For this review, use the dimensioned drawing (mm, ordinates from the lowest corner) and the shaded views. Round coordinates to 2 decimals unless told otherwise and drop trailing zeros. Loops run counter-clockwise (first coordinate to the right, second up) from the corner with the lowest first, then second, coordinate; pieces in that order, holes last. Notation, with made-up numbers: (-13, 39.25) -> (34, 39.25) arc R22 ccw to (34, 69.25) -> close; hole circle Ø3 at (6, 74.25). An arc over 180 degrees is marked (long way). Write each question's results on one line, items separated by ' | '.
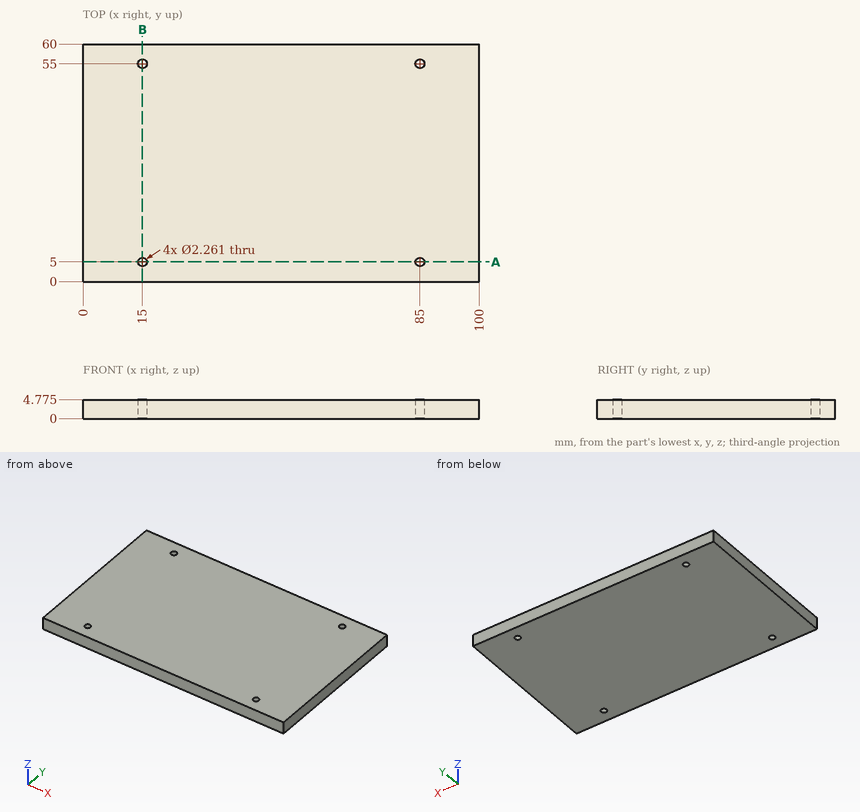
1. Consider section B-B (x = 15). State the section outline as (y, z) points (1 decimal), plus the area to 3 significant figures.
Values found:
outline: (0, 0) -> (3.9, 0) -> (3.9, 4.8) -> (0, 4.8) -> close; (6.1, 0) -> (53.9, 0) -> (53.9, 4.8) -> (6.1, 4.8) -> close; (56.1, 0) -> (60, 0) -> (60, 4.8) -> (56.1, 4.8) -> close | area: 265 mm2
2. To check wall thickness, follow probe 1 along Y at (x, z) = (85, 3.15); probe 2 along X at (y, z) = (4, 1) (1 decimal). State the ranges of each line that lie inside material, in increasing order.
Values found:
probe 1: y = 0 to 3.87, 6.13 to 53.87, 56.13 to 60 | probe 2: x = 0 to 14.5, 15.5 to 84.5, 85.5 to 100
3. Consider section A-A (y = 5). State the section outline as (x, z) points (1 decimal).
Values found:
outline: (0, 0) -> (13.9, 0) -> (13.9, 4.8) -> (0, 4.8) -> close; (16.1, 0) -> (83.9, 0) -> (83.9, 4.8) -> (16.1, 4.8) -> close; (86.1, 0) -> (100, 0) -> (100, 4.8) -> (86.1, 4.8) -> close
4. For pin 1 (1.4 mm diameter, centred on x = 85, y = 55, fed in from +Z), flat-tipped, find the tip position at first contact; note if it passes through.
Values found:
pin 1: passes through
